Design review of the part built by this model. Coordinates are the model's own, in mm. A direction names the side the tool comes from. Give positions to 0.01 mm unless a question says otherwise; leave off trailing zeros. Order: outer loops, then holes, each group sorted by start corner. A loop starts at its lowest first (then second) coordinate and runs counter-clockwise, first axis right, second up. Notation, with made-up numbers: (69, 23.5) -> (115, 23.5) arc R26 ccw to (115, 61.5) -> close; hole circle Ø2 at (17, 40.5). An arc over 180 degrees is marked (long way). Return JSON: item names as keys, results as strings.
```python
from build123d import *

# Parameters (mm, degrees)
F0_W     = 100
F0_H     = 22
F1_DEPTH = 10


with BuildPart() as f1:
    # F0 (on Top) → F1 (new body)
    with BuildSketch(Plane.XY):
        with Locations((11.818181, 1.5)):
            Rectangle(F0_W, F0_H)
        with BuildLine():
            Line((-38.181819, -9.5), (-38.181819, 12.5))
            Line((-38.181819, 12.5), (-38.181819, 16.5))
            ThreePointArc((-38.181819, 16.5), (-53.181819, 1.5), (-38.181819, -13.5))
            Line((-38.181819, -13.5), (-38.181819, -9.5))
        make_face()
        with BuildLine():
            Line((61.818181, 16.5), (61.818181, 12.5))
            Line((61.818181, 12.5), (61.818181, -9.5))
            Line((61.818181, -9.5), (61.818181, -13.5))
            ThreePointArc((61.818181, -13.5), (76.818181, 1.5), (61.818181, 16.5))
        make_face()
    extrude(amount=F1_DEPTH)


solid = f1.part
```
Item 1: Machinability: for faces 1 (the face through (11, 12.5, 5)), 2 (the face through (61.818, -11, 5)), 3 (the face through (11, 2, 0)), which of the approach directions +Z, -Z, +X, -X, +Y, -Y give a long, thin tool a straight path to every point of the face, cutting with its end or side? Answer none if there is none.
Result set:
{"face 1": "+Z, -Z, +Y", "face 2": "+Z, -Z, -Y", "face 3": "-Z, +X, -X, +Y, -Y"}
Item 2: Mouldability with a two-part tool opening along X and no side actions: class faces 4 (the face through (-53.18, 1.83, 4.93)), 5 (the face through (76.815, 1.17, 4.93)), 6 (the face through (61.818, 15, 5)), 7 (the face through (11, 2, 10)) as released by +X, released by -X, zero draft, split by the parting line, or undercut.
Result set:
{"face 4": "released by -X", "face 5": "released by +X", "face 6": "undercut", "face 7": "zero draft"}
Item 3: Wall thickness on L1, parallel to Y at x = 55, z = 3; L2, parallel to Y at x = -38.5, z = 0.75; L3, parallel to X at y = -12, z = 3: over which ranges is each line inside the solid? List them lowest first. Write a range as [from, to].
Result set:
{"L1": "y = [-9.5, 12.5]", "L2": "y = [-13.5, 16.5]", "L3": "x = [-44.72, -38.18], [61.82, 68.36]"}
Item 4: Add section A-A (z = 4.75). Give the boundary of the cut face in (x, y), plus the area to 3 significant figures.
Result set:
{"outline": "(-38.18, -13.5) -> (-38.18, -9.5) -> (61.82, -9.5) -> (61.82, -13.5) arc R15 ccw to (61.82, 16.5) -> (61.82, 12.5) -> (-38.18, 12.5) -> (-38.18, 16.5) arc R15 ccw to start", "area": "2,910 mm^2"}
Item 5: For pin 1 (5 mm diameter, centred on x = 12.5, z = 1, fed in from -Y); pin 2 (1 mm diameter, centred on y = -7, z = 8.5, fed in from +X); pin 3 (3 mm diameter, centred on y = 13.5, z = 3, fed in from -X), all flat-tipped, find the tip position at first contact; note any pin that passes through.
Result set:
{"pin 1": "stops at y = -9.5", "pin 2": "stops at x = 74.51", "pin 3": "stops at x = -48.89"}
Item 6: Add section B-B (x = -3.5). Give the boundary of the cut face in (y, z), plus the area to 3 significant figures.
Result set:
{"outline": "(-9.5, 0) -> (12.5, 0) -> (12.5, 10) -> (-9.5, 10) -> close", "area": "220 mm^2"}
Item 7: Add section C-C (y = -6.5). Give the boundary of the cut face in (x, z).
Result set:
{"outline": "(-50.87, 0) -> (74.51, 0) -> (74.51, 10) -> (-50.87, 10) -> close"}
